from build123d import *

# Parameters (mm, degrees)
F1_DEPTH = 25.4
F2_SIZE  = 12.7
F3_DEPTH = 38.1
F4_SIZE  = 31.7499
F5_SIZE  = 5.08


# Not quite as in the source:
# - a fillet or chamfer is up to 0.001 mm smaller than in the source, because OpenCascade refuses the exact size


with BuildPart() as f1:
    # F0 (on Top) → F1 (new body)
    with BuildSketch(Plane.XY):
        Polygon((31.75, -13.1512806053), (31.75, 13.1512806053), (13.1512806053, 31.75), (-13.1512806053, 31.75), (-31.75, 13.1512806053), (-31.75, -13.1512806053), (-13.1512806053, -31.75), (13.1512806053, -31.75), align=None)
    extrude(amount=F1_DEPTH)

    # F2
    f2_edges = [f1.edges().sort_by_distance(p)[0] for p in [
        (-31.75, 0, 25.4),
        (-22.45064, -22.45064, 25.4),
        (0, -31.75, 25.4),
        (22.45064, -22.45064, 25.4),
        (31.75, 0, 25.4),
        (22.45064, 22.45064, 25.4),
        (0, 31.75, 25.4),
        (-22.45064, 22.45064, 25.4),
    ]]
    chamfer(f2_edges, length=F2_SIZE)

    # F3 (add): a face of the model
    f3_faces = [f1.faces().sort_by_distance(p)[0] for p in [
        (0, 0, 0),
    ]]
    extrude(f3_faces, amount=F3_DEPTH)

    # F4 (size 31.75 in the source; OpenCascade refuses exactly that, so slightly less here)
    f4_edges = [f1.edges().sort_by_distance(p)[0] for p in [
        (-22.45064, -22.45064, -38.1),
        (0, -31.75, -38.1),
        (22.45064, -22.45064, -38.1),
        (-31.75, 0, -38.1),
        (-22.45064, 22.45064, -38.1),
        (0, 31.75, -38.1),
        (22.45064, 22.45064, -38.1),
        (31.75, 0, -38.1),
    ]]
    chamfer(f4_edges, length=F4_SIZE)

    # F5
    f5_edges = [f1.edges().sort_by_distance(p)[0] for p in [
        (-31.75, 0, -6.3501),
        (-22.45064, 22.45064, -6.3501),
        (-22.45064, -22.45064, -6.3501),
        (0, -31.75, -6.3501),
        (22.45064, -22.45064, -6.3501),
        (31.75, 0, -6.3501),
        (22.45064, 22.45064, -6.3501),
        (0, 31.75, -6.3501),
    ]]
    chamfer(f5_edges, length=F5_SIZE)


solid = f1.part
Input: part model. Units: mm. Frame: model coordinates. Give positions to 0.01 mm unless a question says otherwise; leave off trailing zeros. Write each loop counter-clockwise with the first axis right and the second up, starting at its lowest first coordinate (ties: lowest second). Pieces come first, ordered by that corner, then holes. Notation, with made-up numbers: (-14, 84.25) -> (16, 84.25) arc R23 cw to (16, 108.25) -> close; hole circle Ø2 at (77.5, 14.5). An arc over 180 degrees is marked (long way). Use one line per item in the form item = value. Start each with the question number.
1) Pin query (flat end, axial travel): pin 1 (5 mm diameter, centred on x = -11, z = -25, fed in from +Y); pin 2 (5 mm diameter, centred on x = 20.5, z = -9.5, fed in from -Y); pin 3 (1.5 mm diameter, centred on y = -20.5, z = 9, fed in from +X). Return the tip coordinate at first contact, or that it passes through.
2) Section query B-B on y = -18. Return the cut outline in (x, z).
3) Ray query, probe 1 along Z at (x, y) = (3, -8.5); probe 2 along Y at (x, z) = (-4, -28); probe 3 along Y at (x, z) = (1, -5.5). Return the intervals inside material, ascending. Write a range as from..to.
4) Section query A-A on z = 0. Return the cut outline in (x, y).
5) Section query C-C on x = -24. Return the cut outline in (y, z).
6) Section query D-D on y = -2. Return the cut outline in (x, z).
Outcome:
q1.pin_1 = 11.86
q1.pin_2 = -22.48
q1.pin_3 = 25.15
q2.outline = (-26.9, -1.27) -> (-21.82, -9.94) -> (-7.46, -20.1) -> (7.46, -20.1) -> (21.82, -9.94) -> (26.9, -1.27) -> (26.9, 12.7) -> (8.94, 25.4) -> (-8.94, 25.4) -> (-26.9, 12.7) -> close
q3.probe_1 = -29.6..25.4
q3.probe_2 = -10.1..10.1
q3.probe_3 = -30..30
q4.outline = (-31.75, -13.15) -> (-13.15, -31.75) -> (13.15, -31.75) -> (31.75, -13.15) -> (31.75, 13.15) -> (13.15, 31.75) -> (-13.15, 31.75) -> (-31.75, 13.15) -> close
q5.outline = (-20.9, -1.27) -> (-15.82, -9.94) -> (-9.94, -14.1) -> (9.94, -14.1) -> (15.82, -9.94) -> (20.9, -1.27) -> (20.9, 12.7) -> (9.94, 20.45) -> (-9.94, 20.45) -> (-20.9, 12.7) -> close
q6.outline = (-31.75, -1.27) -> (-28.16, -9.94) -> (-4.83, -33.27) -> (-0.83, -36.1) -> (0.83, -36.1) -> (4.83, -33.27) -> (28.16, -9.94) -> (31.75, -1.27) -> (31.75, 12.7) -> (19.05, 25.4) -> (-19.05, 25.4) -> (-31.75, 12.7) -> close
